Source: CAD feature listing. Evaluate the final solid. Frame: model axes, mm. A direction names the side the tool comes from. Coordinates: 2 decimals unless noted, no trailing zeros. Write each loop counter-clockwise with the first axis right and the second up, starting at its lowest first coordinate (ties: lowest second). Pieces come first, ordered by that corner, then holes. Notation, with made-up numbers: M -15,44.5 L -2,44.5 A13 ccw -2,69.5 Z; hole C 74,27.5 d10. An arc over 180 degrees is marked long. One line per item, written item: value. Start each with the question number.
Item 1: Pin query (flat end, axial travel): P1, Ø6.5, axis at x = 2.75, y = 0, coming from the -Z side; P2, Ø4, axis at x = -20.25, y = 0, coming from the -Z side; P3, Ø4, axis at x = -20.25, y = 0, coming from the +Z side. Return the tip coordinate at first contact, or that it passes through.
Item 2: Mould query, pull axis Y, two halves, no side actions, for faces 6 (the flat face through (0, -2, 0)), 7 (the flat face through (0, -10, -9)), 8 (the conical face through (16.01, -0.06, -5.57)). Classes: released by +Y, released by -Y, zero draft, split by the parting line, or undercut.
Item 3: Set-up query: faces 1 (the flat face through (-15.74, 9.49, -16.78)), 2 (the flat face through (-15.25, 0, -17)), 3 (the cylindrical face through (0.365, 0.751, -4.563)), 4 (the flat face through (15.74, -9.49, -16.62)), 5 (the cylindrical face through (21.19, 0.33, -3.52)). Return all of +Z, -Z, +X, -X, +Y, -Y with unobstructed straight access to the full face (end or side cutting, diameter ignored); none if empty.
Item 4: Cut plane B-B, the plane z = -4.5. State how many separate pieces and enclosed holes the cut face has, then the cut area to 3 significant figures.
Item 5: Cut plane D-D, the plane x = -2. Output: boundary loops of the cut face in (y, z).
Item 6: Ray query, L1, parallel to X at y = 5, z = -12.75; L2, parallel to Y at x = 2.75, z = -6.5. Return the intervals inside material, ascending. Write a range as from..to.
Item 7: Cut plane C-C, the plane y = -6.75. Output: boundary loops of the cut face in (x, z), then the cut area to 3 significant figures.
Item 8: Cut plane A-A, the plane x = 11.5. Output: boundary loops of the cut face in (y, z), then the cut area to 3 significant figures.
```python
from build123d import *

# Parameters (mm, degrees)
F1_DEPTH = 10
F3_D     = 5
F3_DEPTH = 8
F3_TIP   = 1.5021515476
F5_D     = 4.2
F5_DEPTH = 9.2
F5_TIP   = 1.2618073
F7_D     = 5
F9_D     = 5
F9_DEPTH = 9
F9_TIP   = 1.5021515476
F10_SIZE = 1
F11_R    = 1


# Not quite as in the source:
# - a feature names something its author has since deleted; it is built from what else it names


with BuildPart() as f1:
    # F0 (on Front) → F1 (new body, symmetric)
    with BuildSketch(Plane.XZ):
        Polygon((-25.25, 0), (-25.25, -22.4), (-15.25, -22.4), (-15.25, -12), (15.25, -12), (15.25, -22.4), (25.25, -22.4), (25.25, 0), align=None)
    extrude(amount=F1_DEPTH, both=True)

    # F3
    with Locations(Plane.YZ.offset(25.25)):
        with Locations((0, -6)):
            Hole(F3_D / 2, depth=F3_DEPTH)
            with Locations((0, 0, -(F3_DEPTH + F3_TIP / 2))):  # 118° drill point
                Cone(0, F3_D / 2, F3_TIP, mode=Mode.SUBTRACT)

    # F5
    with Locations(Plane(origin=(0, 0, -22.4), x_dir=(1, 0, 0), z_dir=(0, 0, -1))):
        with Locations((-20.25, 0), (20.25, 0)):
            Hole(F5_D / 2, depth=F5_DEPTH)
            with Locations((0, 0, -(F5_DEPTH + F5_TIP / 2))):  # 118° drill point
                Cone(0, F5_D / 2, F5_TIP, mode=Mode.SUBTRACT)

    # F7 (through all)
    with Locations(Plane.XZ.offset(10)):
        with Locations((11.5, -6), (-11.5, -6)):
            Hole(F7_D / 2)

    # F9
    with Locations(Plane.XY):
        with Locations((-20.25, 0), (2.75, 0)):
            Hole(F9_D / 2, depth=F9_DEPTH)
            with Locations((0, 0, -(F9_DEPTH + F9_TIP / 2))):  # 118° drill point
                Cone(0, F9_D / 2, F9_TIP, mode=Mode.SUBTRACT)

    # F10
    f10_edges = [f1.edges().sort_by_distance(p)[0] for p in [
        (15.25, 0, -22.4),
        (-15.25, 0, -22.4),
        (-15.25, -10, -17.2),
        (0, -10, -12),
        (15.25, -10, -17.2),
        (0, 10, -12),
        (-15.25, 10, -17.2),
        (15.25, 10, -17.2),
    ]]
    chamfer(f10_edges, length=F10_SIZE)

    # F11
    f11_edges = [f1.edges().sort_by_distance(p)[0] for p in [
        (0, 10, 0),
        (0, -10, 0),
        (-25.25, 0, 0),
        (25.25, 0, 0),
    ]]
    fillet(f11_edges, radius=F11_R)


solid = f1.part
```
From the geometry:
1. P1: stops at z = -12
1. P2: stops at z = -13.14
1. P3: stops at z = -9.3
2. face 6: zero draft
2. face 7: released by -Y
2. face 8: undercut
3. face 1: -Z, +Y
3. face 2: -Z, +Y, -Y
3. face 3: +Z
3. face 4: -Z, -Y
3. face 5: +X
4. separate pieces: 3
4. enclosed holes: 2
4. area: 777 mm²
5. outline: M -10,-11 L -9,-12 L 9,-12 L 10,-11 L 10,-1 A1 ccw 9,0 L -9,0 A1 ccw -10,-1 Z
6. L1: x = -25.25..-15.25, 15.25..25.25
6. L2: y = -10..-2.5, 2.5..10
7. outline: M -25.25,-22.4 L -16.25,-22.4 L -15.25,-21.4 L -15.25,-12 L 15.25,-12 L 15.25,-21.4 L 16.25,-22.4 L 25.25,-22.4 L 25.25,-1 A1 ccw 24.25,0 L -24.25,0 A1 ccw -25.25,-1 Z; hole C -11.5,-6 d5; hole C 11.5,-6 d5
7. area: 773 mm²
8. outline: M -10,-11 L -9,-12 L 9,-12 L 10,-11 L 10,-8.5 L -10,-8.5 Z; M -10,-3.5 L 10,-3.5 L 10,-1 A1 ccw 9,0 L -9,0 A1 ccw -10,-1 Z
8. area: 139 mm²
